CAD build for the part. Positions are in the model's coordinates, mm. A direction names the side the tool comes from. Round coordinates to 2 decimals unless told otherwise and drop trailing zeros. Order: outer loops, then holes, each group sorted by start corner. A loop starts at its lowest first (then second) coordinate and runs counter-clockwise, first axis right, second up. Notation, with made-up numbers: M 59,-10.5 L 75,-10.5 A17 cw 75,-6.5 Z; hole C 71.5,20 d1. An arc over 180 degrees is marked long. Put each result on its own line as item: value.
```python
from build123d import *

# Parameters (mm, degrees)
SKETCH2_R           = 15
BOSS_EXTRUDE3_DEPTH = 100


with BuildPart() as part:
    # Sketch2 → Boss-Extrude3 (new body)
    with BuildSketch(Plane.XY):
        with BuildLine():
            add(Edge.make_bspline(
                [(0, 0), (-27.790971102, 4.850972812), (-43.593467312, 21.015270296), (-47.40748863, 48.492892452)],
                knots=[0, 0, 0, 0, 0.824388571, 0.824388571, 0.824388571, 0.824388571], degree=3))
            Line((0, 0), (0, 12))
            add(Edge.make_bspline(
                [(0, 12), (-19.855506459, 23.701138321), (-2.078921696, 41.432276663)],
                knots=[0, 0, 0, 1, 1, 1], degree=2))
            ThreePointArc((-2.078921696, 41.432276663), (-15.477506866, 78.560495393), (-48.159097141, 56.425898768))
            add(Edge.make_bspline(
                [(-47.40748863, 48.492892452), (-47.761040822, 51.040013382), (-48.011576992, 53.684348821), (-48.159097141, 56.425898768)],
                knots=[0.824388571, 0.824388571, 0.824388571, 0.824388571, 0.900807752, 0.900807752, 0.900807752, 0.900807752], degree=3))
        make_face()
        with Locations((-23.212854475, 54.787308872)):
            Circle(SKETCH2_R, mode=Mode.SUBTRACT)
    extrude(amount=BOSS_EXTRUDE3_DEPTH)


solid = part.part
```
Item 1: Probe line 1 along Y through (x, z) = (-18, 32.5); line 2 along Y through (x, z) = (-16, 24); line 3 along X through (y, z) = (60, 40.5). List the from-to ranges inside material, lowest first. Write a range as [from, to].
Answers below:
line 1: [5.48, 40.72], [68.85, 79.24]
line 2: [4.59, 41.64], [67.94, 78.72]
line 3: [-47.66, -37.28], [-9.15, 1.24]
Item 2: Band-saw the part on A-A on y = 62. Give the cut face in (x, z), and give its area (3 significant figures).
Answers below:
outline: M -47.15,0 L -36.36,0 L -36.36,100 L -47.15,100 Z; M -10.06,0 L 0.72,0 L 0.72,100 L -10.06,100 Z
area: 2,160 mm²
Item 3: Tool access for faces 4 (the flat face through (-17, 40, 0)), 5 (the flat face through (0, 6, 49)): list every direction of +Z, -Z, +X, -X, +Y, -Y with a clear straight run to the whole face (end or side of a thin tool).
Answers below:
face 4: -Z, +X, -X, +Y, -Y
face 5: +Z, -Z, +X, -Y
Item 4: Pin check, flat tips, straight feed: P1, Ø3, axis at x = -10, z = 52, coming from the +Y side; P2, Ø8, axis at x = -9, z = 44.5, coming from the -Y side; P3, Ø1.5, axis at x = -16.5, y = 42.5, coming from the +Z side; P4, Ø6, axis at y = 69.5, z = 58.5, coming from the -X side. Stop position of each tip, or through.
Answers below:
P1: y = 76.87
P2: y = 1.03
P3: through
P4: x = -45.3
Item 5: Mould opens along X. For faces 1 (the flat face through (-17, 40, 100)), 2 (the cylindrical face through (-14.874, 78.356, 49.3)), 3 (the cylindrical face through (-9.357, 49.042, 49.3)) say: pulls with the +X half, pulls with the -X half, needs draft (parallel to the pull), parting line crosses it, or undercut.
Answers below:
face 1: needs draft
face 2: parting line crosses it
face 3: undercut
